Input: part model. Units: mm. Frame: model coordinates. Face numbers are marked on the shaded views. Coordinates: 2 decimals unless noted, no trailing zeros. Write each loop counter-clockwise with the first axis right and the second up, starting at its lowest first coordinate (ties: lowest second). Pieces come first, ordered by that corner, then holes.
from build123d import *

# Parameters (mm, degrees)
F0_R     = 19
F0_R_2   = 3.5
F1_DEPTH = 2
F2_R     = 17.5
F2_R_2   = 3.5
F3_DEPTH = 7
F4_R     = 2
F5_DEPTH = 25


with BuildPart() as f1:
    # F0 (on Top) → F1 (new body)
    with BuildSketch(Plane.XY):
        Circle(F0_R)
        Circle(F0_R_2, mode=Mode.SUBTRACT)
    extrude(amount=F1_DEPTH)

    # F2 (on face) → F3 (join)
    with BuildSketch(Plane.XY.offset(2)):
        Circle(F2_R)
        Circle(F2_R_2, mode=Mode.SUBTRACT)
    extrude(amount=F3_DEPTH)

    # F4 (on face) → F5 (cut)
    with BuildSketch(Plane.XY.offset(9)):
        with Locations((0, 12)):
            Circle(F4_R)
        with Locations((-12, 0)):
            Circle(F4_R)
        with Locations((0, -12)):
            Circle(F4_R)
        with Locations((12, 0)):
            Circle(F4_R)
    extrude(amount=-F5_DEPTH, mode=Mode.SUBTRACT)


solid = f1.part
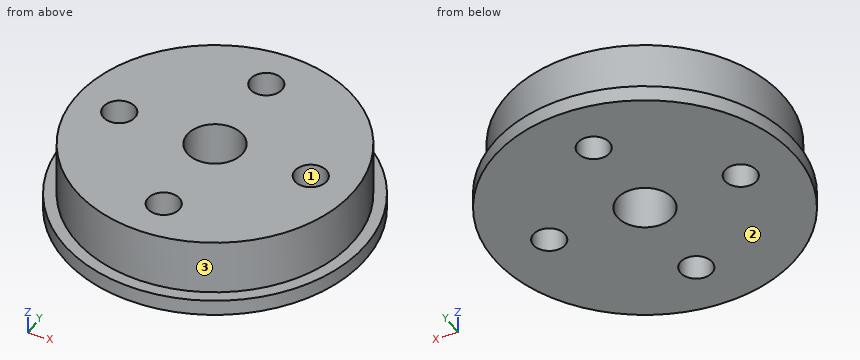
Item 1: Section query D-D, the plane x = 0. Return loops of the section in (y, z).
Item 2: Section query A-A, the plane z = 5.5. Return loops of the section in (x, y).
Item 3: Pin query (flat end, axial travel): pin 1 Ø1 at (x, y) = (5, -12) entering from -Z; pin 2 Ø1 at (y, z) = (1, 7) entering from -X; pin 3 Ø4 at (x, z) = (-12, 1) entering from -Y; pin 4 Ø1 at (y, z) = (10, 6) entering from -X. Return the tip coordinate at first contact, or that it passes through.
Item 4: Section query B-B, the plane x = 10.5. Return loops of the section in (y, z), then the cut area to 3 significant figures.
Item 5: Material intervals for line 1 (Y direction, x = 0, z = 3); line 2 (Y direction, x = 0, z = 1.5); line 3 (Y direction, x = -12, z = 6), sorted ascending.
Item 6: Section query C-C, the plane y = 1.5. Return loops of the section in (x, z), then the cut area to 3 significant figures.
Item 7: Pull-direction query (X, two-part tool) for the marked faces 1, 2 and 3; classes: released by +X, released by -X, zero draft, split by the parting line, or undercut.
The answers:
1. outline: (-19, 0) - (-14, 0) - (-14, 9) - (-17.5, 9) - (-17.5, 2) - (-19, 2) - close; (-10, 0) - (-3.5, 0) - (-3.5, 9) - (-10, 9) - close; (3.5, 0) - (10, 0) - (10, 9) - (3.5, 9) - close; (14, 0) - (19, 0) - (19, 2) - (17.5, 2) - (17.5, 9) - (14, 9) - close
2. outline: circle Ø35 at (0, 0); hole circle Ø4 at (-12, 0); hole circle Ø7 at (0, 0); hole circle Ø4 at (0, -12); hole circle Ø4 at (0, 12); hole circle Ø4 at (12, 0)
3. pin 1: stops at z = 0
3. pin 2: stops at x = -17.49
3. pin 3: stops at y = -16.16
3. pin 4: stops at x = -14.7
4. outline: (-15.84, 0) - (-1.32, 0) - (-1.32, 9) - (-14, 9) - (-14, 2) - (-15.84, 2) - close; (1.32, 0) - (15.84, 0) - (15.84, 2) - (14, 2) - (14, 9) - (1.32, 9) - close
4. area: 236 mm2
5. line 1: y = -17.5 to -14, -10 to -3.5, 3.5 to 10, 14 to 17.5
5. line 2: y = -19 to -14, -10 to -3.5, 3.5 to 10, 14 to 19
5. line 3: y = -12.74 to -2, 2 to 12.74
6. outline: (-18.94, 0) - (-13.32, 0) - (-13.32, 9) - (-17.44, 9) - (-17.44, 2) - (-18.94, 2) - close; (-10.68, 0) - (-3.16, 0) - (-3.16, 9) - (-10.68, 9) - close; (3.16, 0) - (10.68, 0) - (10.68, 9) - (3.16, 9) - close; (13.32, 0) - (18.94, 0) - (18.94, 2) - (17.44, 2) - (17.44, 9) - (13.32, 9) - close
6. area: 215 mm2
7. face 1: undercut
7. face 2: zero draft
7. face 3: split by the parting line
